For this review, take the finished solid that the model builds, in its own axes (mm). Face numbers are marked on the shaded views. A direction names the side the tool comes from. Coordinates: 2 decimals unless noted, no trailing zeros. Write each loop counter-clockwise with the first axis right and the second up, starting at its lowest first coordinate (ties: lowest second). Pieces come first, ordered by that corner, then holes.
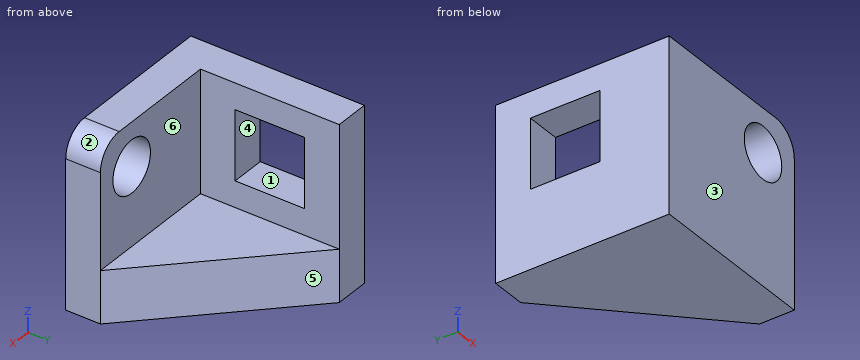
```python
from build123d import *

# Parameters (mm, degrees)
CROQUIS1_W              = 100
CROQUIS1_H              = 100
SALIENTE_EXTRUIR1_DEPTH = 20
CROQUIS2_W              = 20
CROQUIS2_H              = 100
SALIENTE_EXTRUIR2_DEPTH = 80
CROQUIS3_W              = 80
CROQUIS3_H              = 30
SALIENTE_EXTRUIR3_DEPTH = 80
CORTAR_EXTRUIR1_DEPTH   = 80
CROQUIS5_R              = 15
CORTAR_EXTRUIR2_DEPTH   = 80
REDONDEO1_R             = 15
CROQUIS6_W              = 40
CROQUIS6_H              = 40
CORTAR_EXTRUIR3_DEPTH   = 80


with BuildPart() as part:
    # Croquis1 → Saliente-Extruir1 (new body)
    with BuildSketch(Plane(origin=(0, 0, 0), x_dir=(1, 0, 0), z_dir=(0, 1, 0))):
        Rectangle(CROQUIS1_W, CROQUIS1_H)
    extrude(amount=SALIENTE_EXTRUIR1_DEPTH)

    # Croquis2 → Saliente-Extruir2 (add)
    with BuildSketch(Plane(origin=(0, 20, 0), x_dir=(1, 0, 0), z_dir=(0, 1, 0))):
        with Locations((-40, 0)):
            Rectangle(CROQUIS2_W, CROQUIS2_H)
    extrude(amount=SALIENTE_EXTRUIR2_DEPTH)

    # Croquis3 → Saliente-Extruir3 (add)
    with BuildSketch(Plane(origin=(0, 20, 0), x_dir=(1, 0, 0), z_dir=(0, 1, 0))):
        with Locations((10, 35)):
            Rectangle(CROQUIS3_W, CROQUIS3_H)
    extrude(amount=SALIENTE_EXTRUIR3_DEPTH)

    # Croquis4 → Cortar-Extruir1 (cut)
    with BuildSketch(Plane.XY.offset(-20)):
        Polygon((50, 20), (-30, 100), (50, 100), align=None)
    extrude(amount=-CORTAR_EXTRUIR1_DEPTH, mode=Mode.SUBTRACT)

    # Croquis5 → Cortar-Extruir2 (cut)
    with BuildSketch(Plane(origin=(0, 20, 0), x_dir=(1, 0, 0), z_dir=(0, 1, 0))):
        with Locations((25, -25)):
            Circle(CROQUIS5_R)
    extrude(amount=-CORTAR_EXTRUIR2_DEPTH, mode=Mode.SUBTRACT)

    # Redondeo1
    redondeo1_edges = [part.edges().sort_by_distance(p)[0] for p in [
        (50, 10, 50),
    ]]
    fillet(redondeo1_edges, radius=REDONDEO1_R)

    # Croquis6 → Cortar-Extruir3 (cut)
    with BuildSketch(Plane(origin=(-30, 0, 0), x_dir=(0, 0, -1), z_dir=(1, 0, 0))):
        with Locations((-15, 60)):
            Rectangle(CROQUIS6_W, CROQUIS6_H)
    extrude(amount=-CORTAR_EXTRUIR3_DEPTH, mode=Mode.SUBTRACT)


solid = part.part
```
1) Consider section A-A (y = 45). Give the boundary of the cut face in (x, z), then the cut area to 3 significant figures.
2) For L1, parallel to Z at x = 25, y = 12.5; L2, parallel to Y at x = -34.5, z = 14.5, list the stretches that pass through material, from the lowest coordinate up.
3) Consider section B-B (z = 25). Give the boundary of the cut face in (x, y), then the cut area to 3 significant figures.
4) The part is to be moulded in two halves that separate along Y. For the marked faces 1, 2 and 3, say which applies: pulls with the +Y half, pulls with the -Y half, needs draft (parallel to the pull), parting line crosses it, or undercut.
5) Consider section C-C (x = 25). Give the boundary of the cut face in (y, z), then the cut area to 3 significant figures.
6) Clearance check with flat-ended pins moving along their axes: P1, Ø1.5, axis at y = 75, z = -26.5, coming from the +X side; P2, Ø10, axis at x = -39, z = 7, coming from the -Y side; P3, Ø6, axis at x = -13, z = -25.5, coming from the +Y side; P4, Ø6, axis at x = -14.5, y = 47, coming from the +Z side. State where each tip first meets the part, or that it passes through.
7) Tool access review of the marked faces 4, 5 and 6: name each direction out of +Z, -Z, +X, -X, +Y, -Y from which nothing blocks a thin tool from reaching the whole face with its end or side.
8) Consider section D-D (x = -22). Give the boundary of the cut face in (y, z), then the cut area to 3 significant figures.
Results:
1. outline: (-50, -50) - (25, -50) - (25, -20) - (-30, -20) - (-30, -5) - (-50, -5) - close; (-50, 35) - (-30, 35) - (-30, 50) - (-50, 50) - close
1. area: 2,850 mm2
2. L1: z = -50 to 10, 40 to 50
2. L2: y = 0 to 40, 80 to 100
3. outline: (-50, 0) - (10, 0) - (10, 20) - (-30, 20) - (-30, 40) - (-50, 40) - close; (-50, 80) - (-30, 80) - (-30, 100) - (-50, 100) - close; (40, 0) - (50, 0) - (50, 20) - (40, 20) - close
3. area: 2,200 mm2
4. face 1: undercut
4. face 2: needs draft
4. face 3: pulls with the -Y half
5. outline: (0, -50) - (45, -50) - (45, -20) - (20, -20) - (20, 10) - (0, 10) - close; (0, 40) - (20, 40) - (20, 50) - (0, 50) - close
5. area: 2,150 mm2
6. P1: stops at x = -4.25
6. P2: stops at y = 0
6. P3: stops at y = 86
6. P4: stops at z = -20
7. face 4: +X, -X
7. face 5: +Z, -Z, +X, +Y
7. face 6: +Z, +X, +Y
8. outline: (0, -50) - (92, -50) - (92, -20) - (20, -20) - (20, 50) - (0, 50) - close
8. area: 4,160 mm2
